```python
from build123d import *

# Parameters (mm, degrees)
F1_DEPTH = 10
F3_D     = 5
F3_DEPTH = 5
F3_TIP   = 1.5021515476
F5_D     = 1
F5_DEPTH = 5
F5_TIP   = 0.3004303095
F6_R     = 5


with BuildPart() as f1:
    # F0 (on Top) → F1 (new body)
    with BuildSketch(Plane.XY):
        with BuildLine():
            Line((-110, 0), (-5, 0))
            ThreePointArc((-5, 0), (-8.5355339059, 8.5355339059), (0, 5))
            Line((0, 5), (0, 95))
            ThreePointArc((0, 95), (-8.5355339059, 91.4644660941), (-5, 100))
            Line((-5, 100), (-110, 100))
            ThreePointArc((-110, 100), (-138.2842712475, 88.2842712475), (-150, 60))
            Line((-150, 60), (-150, 40))
            ThreePointArc((-150, 40), (-138.2842712475, 11.7157287525), (-110, 0))
        make_face()
    extrude(amount=F1_DEPTH)

    # F3
    with Locations(Plane(origin=(0, 0, 0), x_dir=(1, 0, 0), z_dir=(0, 0, -1))):
        with Locations((-30, -10), (-30, -90)):
            Hole(F3_D / 2, depth=F3_DEPTH)
            with Locations((0, 0, -(F3_DEPTH + F3_TIP / 2))):  # 118° drill point
                Cone(0, F3_D / 2, F3_TIP, mode=Mode.SUBTRACT)

    # F5
    with Locations(Plane(origin=(0, 0, 0), x_dir=(1, 0, 0), z_dir=(0, 0, -1))):
        with Locations((-138.2842712475, -40), (-138.2842712475, -60)):
            Hole(F5_D / 2, depth=F5_DEPTH)
            with Locations((0, 0, -(F5_DEPTH + F5_TIP / 2))):  # 118° drill point
                Cone(0, F5_D / 2, F5_TIP, mode=Mode.SUBTRACT)

    # F6
    f6_edges = [f1.edges().sort_by_distance(p)[0] for p in [
        (-57.5, 100, 10),
        (0, 50, 10),
    ]]
    fillet(f6_edges, radius=F6_R)


solid = f1.part
```
Verification items for the finished model (mm, model axes). A direction names the side the tool comes from. Give positions to 0.01 mm unless a question says otherwise; leave off trailing zeros. One line per item, written item: value.
(1) Tool access check on faces 4 (the face through (-76, 51, 0)), 5 (the face through (-29.46, 12.44, 2.54)). Record the directions out of +Z, -Z, +X, -X, +Y, -Y that give a thin tool (end or side, any length) a straight path to the whole face; none if there is none.
Final values:
face 4: -Z, +X, -X, +Y, -Y
face 5: -Z
(2) Scan lines: line 1 along X through (y, z) = (9.5, 6); line 2 along Y through (x, z) = (-8, 7.25); line 3 along Y through (x, z) = (-5, 6.5). Record each from-to range of solid material in increasing order. Write a range as [from, to].
Final values:
line 1: [-135.72, -30.67], [-29.33, -7.18], [-2.82, -0.1]
line 2: [0.53, 1], [9, 91], [99, 99.47]
line 3: [10, 90]
(3) Draft check along X on faces 1 (the face through (-148, 50, 9)), 2 (the face through (-57, 2, 9)), 3 (the face through (-8, 91, 5)). Enter one of: pulls with the +X half, pulls with the -X half, needs draft (parallel to the pull), parting line crosses it, or undercut.
Final values:
face 1: pulls with the -X half
face 2: needs draft
face 3: undercut
(4) Gauge pin test, flat ends, axial feed: pin 1 (1 mm diameter, centred on y = 23, z = 7, fed in from +X); pin 2 (1.5 mm diameter, centred on y = 50.5, z = 8, fed in from +X); pin 3 (1 mm diameter, centred on x = -132.5, z = 6.5, fed in from -Y). Record the tip position at first contact, or that the pin passes through.
Final values:
pin 1: x = -0.23
pin 2: x = -0.53
pin 3: y = 6.83
